Geometry: see drawing. Coordinates: mm, zero at the bounding-box minimum. Give positions to 0.01 mm unless a question says otherwise; leave off trailing zeros. Order: outer loops, then holes, each group sorted by start corner. A loop starts at its lowest first (then second) coordinate and runs counter-clockwise, first axis right, second up. Notation, with made-up numbers: (18, 56) - (63, 56) arc R18 ccw to (63, 82) - close; hole circle Ø6 at (-3, -28.5). An arc over 180 degrees is marked (long way). One line per question, with ' | ' between items. Start each with the question number.
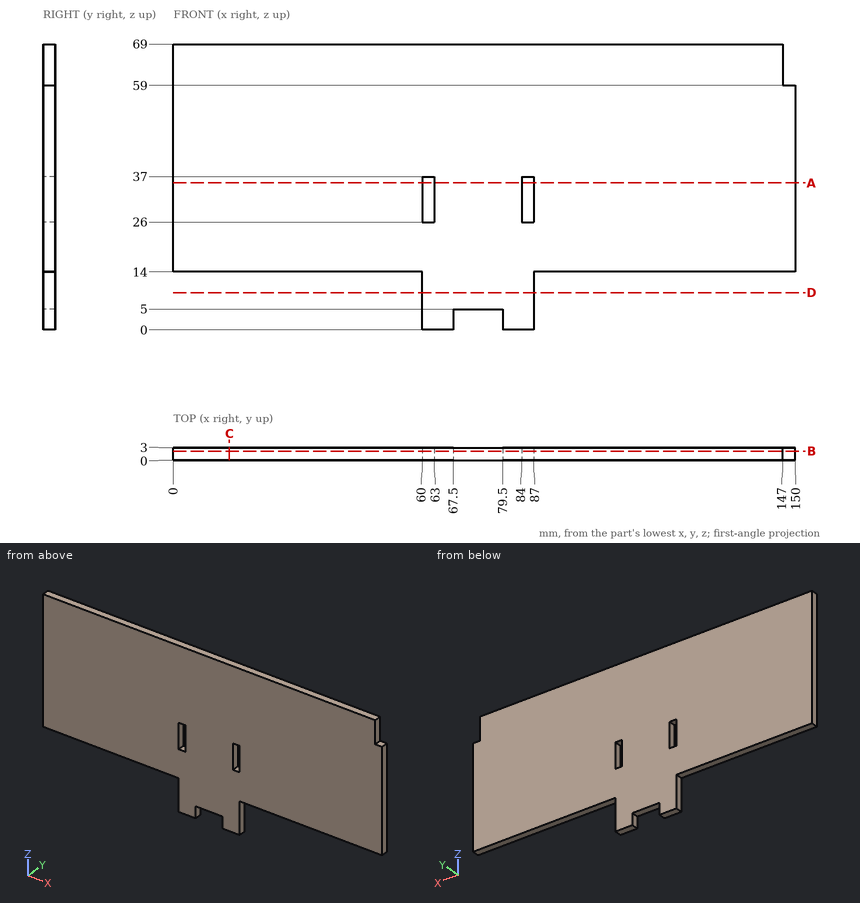
(1) Cut plane B-B, the plane y = 2.2. Return the cut outline in (x, z), plus the area to 3 significant figures.
(2) Cut plane C-C, the plane x = 13.5. Return the cut outline in (y, z).
(3) Cut plane D-D, the plane z = 9. Return the cut outline in (x, y).
(4) Cut plane A-A, the plane z = 35.5. Return the cut outline in (x, y).
(5) Material intervals for line 1 along X through (y, z) = (1.5, 29.5); line 2 along Z through (x, y) = (58.5, 0.9); line 3 along X through (y, z) = (0.8, 62), sorted ascending. Write a range as from..to.
(6) Contact query for flat-ended pins moving along their axis: P1, Ø0.9, axis at x = 149, y = 2, coming from the +Z side; P2, Ø0.9, axis at x = 75, y = 1, coming from the -Z side; P3, Ø1.5, axis at x = 121.5, y = 2.5, coming from the -Z side. Output: stop coordinate, or through.
Results are:
1) outline: (0, 14) - (60, 14) - (60, 0) - (67.5, 0) - (67.5, 5) - (79.5, 5) - (79.5, 0) - (87, 0) - (87, 14) - (150, 14) - (150, 59) - (147, 59) - (147, 69) - (0, 69) - close; hole (60, 26) - (63, 26) - (63, 37) - (60, 37) - close; hole (84, 26) - (87, 26) - (87, 37) - (84, 37) - close | area: 8,470 mm2
2) outline: (0, 14) - (3, 14) - (3, 69) - (0, 69) - close
3) outline: (60, 0) - (87, 0) - (87, 3) - (60, 3) - close
4) outline: (0, 0) - (60, 0) - (60, 3) - (0, 3) - close; (63, 0) - (84, 0) - (84, 3) - (63, 3) - close; (87, 0) - (150, 0) - (150, 3) - (87, 3) - close
5) line 1: 0..60, 63..84, 87..150 | line 2: 14..69 | line 3: 0..147
6) P1: z = 59 | P2: z = 5 | P3: z = 14
